Geometry: final body of the model. Coordinates: model frame, mm. Coordinates: 2 decimals unless noted, no trailing zeros. Write each loop counter-clockwise with the first axis right and the second up, starting at its lowest first coordinate (ties: lowest second). Pieces come first, ordered by that corner, then holes. Notation, with made-up numbers: (78.25, -36.75) -> (133.25, -36.75) arc R19 ccw to (133.25, -17.75) -> close; hole circle Ø11 at (35.5, -25). An arc over 180 degrees is marked (long way). Answer as a JSON object with one key per item and string values. Group by question number.
```python
from build123d import *

# Parameters (mm, degrees)
SKETCH1_W               = 390.8
SKETCH1_H               = 133.8
BOSS_EXTRUDE1_DEPTH     = 6
SKETCH2_W               = 364
SKETCH2_H               = 125.6
CUT_EXTRUDE1_DEPTH      = 5.5
BOSS_EXTRUDE3_DEPTH     = 390.8
SKETCH8_W               = 9.2
SKETCH8_H               = 3.5
CUT_EXTRUDE2_DEPTH      = 10
BOSS_EXTRUDE4_DEPTH     = 5.5
SKETCH11_W              = 15.2
SKETCH11_H              = 5.5
CUT_EXTRUDE3_DEPTH      = 1.5
CUT_EXTRUDE6_DEPTH      = 414.309625425
CUT_EXTRUDE6_DEPTH_BACK = 414.309625425
FILLET1_R               = 4
M2_CLEARANCE_HOLE1_D    = 2.4
CUT_EXTRUDE7_START      = -3
SKETCH13_R              = 2.5
CUT_EXTRUDE7_DEPTH      = 411.496043655
FILLET2_R               = 4


with BuildPart() as part:
    # Sketch1 → Boss-Extrude1 (new body)
    with BuildSketch(Plane(origin=(0, 0, 0), x_dir=(1, 0, 0), z_dir=(0, 1, 0))):
        with Locations((195.4, 66.9)):
            Rectangle(SKETCH1_W, SKETCH1_H)
    extrude(amount=BOSS_EXTRUDE1_DEPTH)

    # Sketch2 → Cut-Extrude1 (cut)
    with BuildSketch(Plane(origin=(0, 6, 0), x_dir=(1, 0, 0), z_dir=(0, 1, 0))):
        with Locations((195.4, 68.1)):
            Rectangle(SKETCH2_W, SKETCH2_H)
    extrude(amount=-CUT_EXTRUDE1_DEPTH, mode=Mode.SUBTRACT)

    # Boss-Extrude3: read off the stored shape, not the designer's step
    # Boss-Extrude3 outline → Boss-Extrude3 (add)
    with BuildSketch(Plane.YZ):
        Polygon((-14.062946679, -133.8), (0, -133.8), (0, 0), align=None)
    extrude(amount=BOSS_EXTRUDE3_DEPTH)

    # Sketch8 → Cut-Extrude2 (cut)
    with BuildSketch(Plane(origin=(0, 0, -133.8), x_dir=(-1, 0, 0), z_dir=(0, 0, -1))):
        with Locations((-34.3, 4.25)):
            Rectangle(SKETCH8_W, SKETCH8_H)
    extrude(amount=-CUT_EXTRUDE2_DEPTH, mode=Mode.SUBTRACT)

    # Sketch10 → Boss-Extrude4 (add)
    with BuildSketch(Plane(origin=(0, 0.5, 0), x_dir=(1, 0, 0), z_dir=(0, 1, 0))):
        with BuildLine():
            Line((99.5, 5.3), (105.5, 5.3))
            ThreePointArc((105.5, 5.3), (102.5, 8.3), (99.5, 5.3))
        make_face()
        with BuildLine():
            ThreePointArc((290.5, 5.3), (287.5, 8.3), (284.5, 5.3))
            Line((284.5, 5.3), (290.5, 5.3))
        make_face()
        with BuildLine():
            Line((105.5, 130.9), (99.5, 130.9))
            ThreePointArc((99.5, 130.9), (102.5, 127.9), (105.5, 130.9))
        make_face()
        with BuildLine():
            ThreePointArc((284.5, 130.9), (287.5, 127.9), (290.5, 130.9))
            Line((290.5, 130.9), (284.5, 130.9))
        make_face()
        with BuildLine():
            Line((198.4, 130.9), (192.4, 130.9))
            ThreePointArc((192.4, 130.9), (195.4, 127.9), (198.4, 130.9))
        make_face()
    extrude(amount=BOSS_EXTRUDE4_DEPTH)

    # Sketch11 → Cut-Extrude3 (cut)
    with BuildSketch(Plane(origin=(0, 0, -133.8), x_dir=(-1, 0, 0), z_dir=(0, 0, -1))):
        with Locations((-34.3, 3.25)):
            Rectangle(SKETCH11_W, SKETCH11_H)
    extrude(amount=-CUT_EXTRUDE3_DEPTH, mode=Mode.SUBTRACT)

    # Sketch12 → Cut-Extrude6 (cut, two sides: drawn at the far end of the back side and taken through both)
    with BuildSketch(Plane.ZY.offset(-CUT_EXTRUDE6_DEPTH_BACK)):
        Polygon((-133.8, -14.062946679), (-121.393278428, -12.758947696), (-133.8, -0.352226124), align=None)
    extrude(amount=CUT_EXTRUDE6_DEPTH + CUT_EXTRUDE6_DEPTH_BACK, mode=Mode.SUBTRACT)

    # Fillet1
    fillet1_edges = [part.edges().sort_by_distance(p)[0] for p in [
        (13.4, 3.25, -5.3),
        (13.4, 3.25, -130.9),
        (377.4, 3.25, -130.9),
        (377.4, 3.25, -5.3),
        (99.5, 3.25, -130.9),
        (105.5, 3.25, -130.9),
        (192.4, 3.25, -130.9),
        (198.4, 3.25, -130.9),
        (284.5, 3.25, -130.9),
        (290.5, 3.25, -130.9),
        (290.5, 3.25, -5.3),
        (284.5, 3.25, -5.3),
        (105.5, 3.25, -5.3),
        (99.5, 3.25, -5.3),
    ]]
    fillet(fillet1_edges, radius=FILLET1_R)

    # M2 Clearance Hole1 (through all)
    with Locations(Plane(origin=(102.5, 6, -5.3), x_dir=(0, 0, 1), z_dir=(0, 1, 0))):
        with Locations((0, 0), (-39.7, -97.2), (-83.5, -97.2), (-125.6, 0), (-125.6, 92.9), (-125.6, 185), (-83.5, 283), (-39.7, 283), (0, 185)):
            Hole(M2_CLEARANCE_HOLE1_D / 2)

    # Sketch13 → Cut-Extrude7 (cut, through all)
    with BuildSketch(Plane(origin=(0, 6, 0), x_dir=(1, 0, 0), z_dir=(0, 1, 0)).offset(CUT_EXTRUDE7_START)):
        with Locations(Location((5.3, 45, 0), (0, 0, 270))):
            Circle(SKETCH13_R)
        with Locations(Location((5.3, 88.8, 0), (0, 0, 270))):
            Circle(SKETCH13_R)
        with Locations(Location((102.5, 5.3, 0), (0, 0, 270))):
            Circle(SKETCH13_R)
        with Locations(Location((287.5, 5.3, 0), (0, 0, 270))):
            Circle(SKETCH13_R)
        with Locations(Location((385.5, 45, 0), (0, 0, 270))):
            Circle(SKETCH13_R)
        with Locations(Location((385.5, 88.8, 0), (0, 0, 270))):
            Circle(SKETCH13_R)
        with Locations(Location((287.5, 130.9, 0), (0, 0, 270))):
            Circle(SKETCH13_R)
        with Locations(Location((195.4, 130.9, 0), (0, 0, 270))):
            Circle(SKETCH13_R)
        with Locations(Location((102.5, 130.9, 0), (0, 0, 270))):
            Circle(SKETCH13_R)
    extrude(amount=-CUT_EXTRUDE7_DEPTH, mode=Mode.SUBTRACT)

    # Fillet2
    # the kernel refuses this fillet: 4 mm, written as the material it adds along each edge
    with BuildSketch(Plane(origin=(41.9, -7.306247498, -132.3), x_dir=(-1, 0, 0), z_dir=(0, 1, 0))) as fillet2_piece_1_section:
        with BuildLine():
            CenterArc((3.122498999, -4), FILLET2_R, 90, 51.317812547)
            Line((0, -1.5), (0, 0))
            Line((0, 0), (3.122498999, 0))
        make_face()
    fillet2_piece_1 = extrude(amount=21.112494996, mode=Mode.PRIVATE)
    fillet2_piece_1 = split(fillet2_piece_1, bisect_by=Plane(origin=(41.9, 2.5, -132.3), z_dir=(0, -1, 0)), keep=Keep.TOP, mode=Mode.PRIVATE)
    fillet2_piece_1 = split(fillet2_piece_1, bisect_by=Plane(origin=(41.9, -4.579236811, -129.572989313), z_dir=(0, 0.7071067811865451, 0.70710678118655)), keep=Keep.TOP, mode=Mode.PRIVATE)
    add(fillet2_piece_1)
    with BuildSketch(Plane(origin=(41.9, -7.306247498, -132.3), x_dir=(-1, 0, 0), z_dir=(0, 1, 0))) as fillet2_piece_2_section:
        with BuildLine():
            CenterArc((3.122498999, -4), FILLET2_R, 90, 51.317812547)
            Line((0, -1.5), (0, 0))
            Line((0, 0), (3.122498999, 0))
        make_face()
    fillet2_piece_2 = extrude(amount=13.306247498, mode=Mode.PRIVATE)
    fillet2_piece_2 = split(fillet2_piece_2, bisect_by=Plane(origin=(38.9, -7.306247498, -132.3), z_dir=(1, 0, 0)), keep=Keep.TOP, mode=Mode.PRIVATE)
    fillet2_piece_2 = split(fillet2_piece_2, bisect_by=Plane(origin=(41.9, -4.579236811, -129.572989313), z_dir=(0, 0.7071067811865451, 0.70710678118655)), keep=Keep.TOP, mode=Mode.PRIVATE)
    add(fillet2_piece_2)
    with BuildSketch(Plane(origin=(26.7, 6, -132.3), x_dir=(1, 0, 0), z_dir=(0, -1, 0))) as fillet2_piece_3_section:
        with BuildLine():
            CenterArc((3.122498999, -4), FILLET2_R, 90, 51.317812547)
            Line((0, -1.5), (0, 0))
            Line((0, 0), (3.122498999, 0))
        make_face()
    fillet2_piece_3 = extrude(amount=13.306247498, mode=Mode.PRIVATE)
    fillet2_piece_3 = split(fillet2_piece_3, bisect_by=Plane(origin=(29.7, 6, -132.3), z_dir=(-1, 0, 0)), keep=Keep.TOP, mode=Mode.PRIVATE)
    fillet2_piece_3 = split(fillet2_piece_3, bisect_by=Plane(origin=(26.7, 2.073886938, -136.226113062), z_dir=(0, 0.7071067811865451, 0.70710678118655)), keep=Keep.TOP, mode=Mode.PRIVATE)
    add(fillet2_piece_3)
    with BuildSketch(Plane(origin=(26.7, 13.806247498, -132.3), x_dir=(1, 0, 0), z_dir=(0, -1, 0))) as fillet2_piece_4_section:
        with BuildLine():
            CenterArc((3.122498999, -4), FILLET2_R, 90, 51.317812547)
            Line((0, -1.5), (0, 0))
            Line((0, 0), (3.122498999, 0))
        make_face()
    fillet2_piece_4 = extrude(amount=21.112494996, mode=Mode.PRIVATE)
    fillet2_piece_4 = split(fillet2_piece_4, bisect_by=Plane(origin=(26.7, 2.5, -132.3), z_dir=(0, -1, 0)), keep=Keep.TOP, mode=Mode.PRIVATE)
    fillet2_piece_4 = split(fillet2_piece_4, bisect_by=Plane(origin=(26.7, 5.977010687, -140.129236811), z_dir=(0, 0.7071067811865451, 0.70710678118655)), keep=Keep.TOP, mode=Mode.PRIVATE)
    add(fillet2_piece_4)


solid = part.part
```
Item 1: Section A-A on x = 165. Output: boundary loops of the cut face in (y, z).
Item 2: Contact query for flat-ended pins moving along their axis: pin 1 (12 mm diameter, centred on x = 260.5, z = -20, fed in from -Y); pin 2 (4 mm diameter, centred on x = 5.3, z = -88.8, fed in from +Y); pin 3 (3 mm diameter, centred on x = 260.5, y = -7, fed in from -Z); pin 4 (3 mm diameter, centred on x = 287.5, z = -130.9, fed in from -Y). Output: stop coordinate, or through.
Item 3: Ray query, L1, parallel to X at y = 4.65, z = -45; L2, parallel to Z at x = 385.5, y = 5; L3, parallel to X at y = 0, z = -130.9. Return the intervals inside material, ascending. Write a range as [from, to].
Item 4: Mould query, pull axis Z, two halves, no side actions, for faces 1 (the flat face through (390.8, -1, -81)), 2 (the flat face through (192.66, -6.29, -59.85)), 3 (the flat face through (193, 0.5, -69)). Classes: +Z half, -Z half, draft (parallel to the pull), parting line (faces both ways), or undercut.
Item 5: Section B-B on z = -63. Output: boundary loops of the cut face in (x, y).
Item 6: Section C-C on z = -117. Output: boundary loops of the cut face in (x, y).
Answer sheet:
{
 "1": {"outline": "(-12.76, -121.39) -> (-0.35, -133.8) -> (6, -133.8) -> (6, -130.9) -> (0.5, -130.9) -> (0.5, -5.3) -> (6, -5.3) -> (6, 0) -> (0, 0) -> close"},
 "2": {"pin 1": "stops at y = -2.73", "pin 2": "stops at y = 6", "pin 3": "stops at z = -128.65", "pin 4": "stops at y = 3"},
 "3": {"L1": "x = [0, 4.1], [6.5, 13.4], [377.4, 384.3], [386.7, 390.8]", "L2": "z = [-133.8, -90], [-87.6, -46.2], [-43.8, 0]", "L3": "x = [0, 100], [105, 192.9], [197.9, 285], [290, 390.8]"},
 "4": {"face 1": "draft", "face 2": "+Z half", "face 3": "undercut"},
 "5": {"outline": "(0, -6.62) -> (390.8, -6.62) -> (390.8, 6) -> (377.4, 6) -> (377.4, 0.5) -> (13.4, 0.5) -> (13.4, 6) -> (0, 6) -> close"},
 "6": {"outline": "(0, -12.3) -> (390.8, -12.3) -> (390.8, 6) -> (377.4, 6) -> (377.4, 0.5) -> (13.4, 0.5) -> (13.4, 6) -> (0, 6) -> close"}
}
